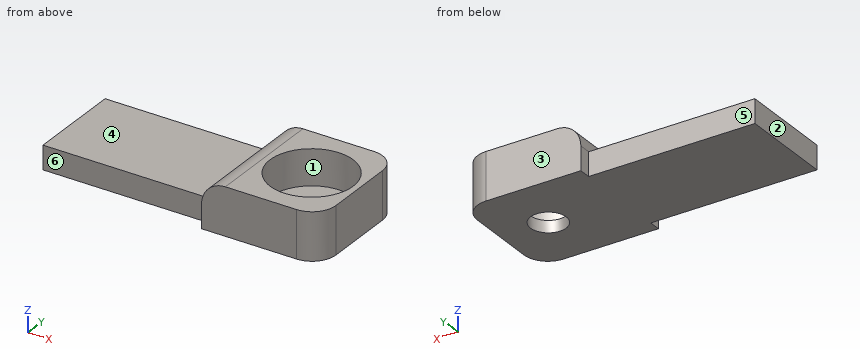
```python
from build123d import *

# Parameters (mm, degrees)
BOSS_EXTRUDE1_DEPTH = 20
CUT_EXTRUDE1_REACH  = 78.974
SKETCH2_R           = 7.5
SKETCH3_R           = 17.5
CUT_EXTRUDE2_DEPTH  = 15
SKETCH4_W           = 10
SKETCH4_H           = 40
CUT_EXTRUDE3_DEPTH  = 70
FILLET1_R           = 10
FILLET2_START       = -26
FILLET2_DEPTH       = 52


with BuildPart() as part:
    # Sketch1 → Boss-Extrude1 (new body)
    with BuildSketch(Plane.XY):
        Polygon((-70, 20), (0, 20), (0, 25), (50, 25), (50, -25), (0, -25), (0, -20), (-70, -20), align=None)
    extrude(amount=BOSS_EXTRUDE1_DEPTH)

    # Sketch2 → Cut-Extrude1 (cut, up to next)
    with BuildSketch(Plane.XY.offset(20), mode=Mode.PRIVATE) as cut_extrude1_sk1:
        with Locations((30, 0)):
            Circle(SKETCH2_R)
    cut_extrude1_tool1 = extrude(cut_extrude1_sk1.sketch, amount=-CUT_EXTRUDE1_REACH, mode=Mode.PRIVATE) & part.part
    add(cut_extrude1_tool1.solids().sort_by_distance((30, 0, 20))[0], mode=Mode.SUBTRACT)

    # Sketch3 → Cut-Extrude2 (cut)
    with BuildSketch(Plane.XY.offset(20)):
        with Locations((30, 0)):
            Circle(SKETCH3_R)
    extrude(amount=-CUT_EXTRUDE2_DEPTH, mode=Mode.SUBTRACT)

    # Sketch4 → Cut-Extrude3 (cut)
    with BuildSketch(Plane.ZY.offset(70)):
        with Locations((15, 0)):
            Rectangle(SKETCH4_W, SKETCH4_H)
    extrude(amount=-CUT_EXTRUDE3_DEPTH, mode=Mode.SUBTRACT)

    # Fillet1
    fillet1_edges = [part.edges().sort_by_distance(p)[0] for p in [
        (50, 25, 10),
        (50, -25, 10),
    ]]
    fillet(fillet1_edges, radius=FILLET1_R)

    # Fillet2: read off the stored shape, not the designer's step
    # Fillet2 outline → Fillet2 (cut)
    with BuildSketch(Plane(origin=(0, 0, 0), x_dir=(1, 0, 0), z_dir=(0, 1, 0)).offset(FILLET2_START)):
        with BuildLine():
            ThreePointArc((10, -20), (2.928932188, -17.071067812), (0, -10))
            Line((0, -10), (0, -20))
            Line((0, -20), (10, -20))
        make_face()
    extrude(amount=FILLET2_DEPTH, mode=Mode.SUBTRACT)


solid = part.part
```
Verification items for the finished model (mm, model axes). Face numbers are marked on the shaded views. A direction names the side the tool comes from. Give positions to 0.01 mm unless a question says otherwise; leave off trailing zeros. Order: outer loops, then holes, each group sorted by start corner. A loop starts at its lowest first (then second) coordinate and runs counter-clockwise, first axis right, second up. Notation, with made-up numbers: (21.25, 46.25) -> (58.25, 46.25) arc R23 ccw to (58.25, 67.25) -> close; hole circle Ø1 at (56, -16.75). An arc over 180 degrees is marked (long way). Use a Markdown table: item, result.
1) Tool access check on the marked faces 4, 5 and 6. Record the directions out of +Z, -Z, +X, -X, +Y, -Y that give a thin tool (end or side, any length) a straight path to the whole face; none if there is none.
Results:
| item | result |
|---|---|
| face 4 | +Z, -X, +Y, -Y |
| face 5 | +Z, -Z, -X, +Y |
| face 6 | +Z, -Z, -X, -Y |
2) Section check D-D, the plane x = 14.5. Record the boundary of the cut face in (y, z).
Results:
| item | result |
|---|---|
| outline | (-25, 0) -> (25, 0) -> (25, 20) -> (8.12, 20) -> (8.12, 5) -> (-8.12, 5) -> (-8.12, 20) -> (-25, 20) -> close |
3) Mould release check, pull along X, two halves, no side actions. Record for the marked faces 1, 2 and 3: pulls with the +X half, pulls with the -X half, needs draft (parallel to the pull), parting line crosses it, or undercut.
Results:
| item | result |
|---|---|
| face 1 | undercut |
| face 2 | pulls with the -X half |
| face 3 | needs draft |
4) Section check C-C, the plane x = 30. Record the boundary of the cut face in (y, z).
Results:
| item | result |
|---|---|
| outline | (-25, 0) -> (-7.5, 0) -> (-7.5, 5) -> (-17.5, 5) -> (-17.5, 20) -> (-25, 20) -> close; (7.5, 0) -> (25, 0) -> (25, 20) -> (17.5, 20) -> (17.5, 5) -> (7.5, 5) -> close |
5) Depth check by flat-ended pin: pin 1 Ø3 at (x, z) = (-46, 4) entering from +Y; pin 2 Ø1.5 at (y, z) = (-23, 4.5) entering from -X; pin 3 Ø19.5 at (x, y) = (30, 0) entering from +Z; pin 4 Ø8 at (x, z) = (-28, 16.5) entering from +Y. Enter the tip coordinate at first touch or a pass-through.
Results:
| item | result |
|---|---|
| pin 1 | y = 20 |
| pin 2 | x = 0 |
| pin 3 | z = 5 |
| pin 4 | through |
6) Section check B-B, the plane y = 0. Record the boundary of the cut face in (x, z).
Results:
| item | result |
|---|---|
| outline | (-70, 0) -> (22.5, 0) -> (22.5, 5) -> (12.5, 5) -> (12.5, 20) -> (10, 20) arc R10 ccw to (0, 10) -> (-70, 10) -> close; (37.5, 0) -> (50, 0) -> (50, 20) -> (47.5, 20) -> (47.5, 5) -> (37.5, 5) -> close |
7) Section check A-A, the plane z = 2.5. Record the boundary of the cut face in (x, y), then the cut area to 3 significant figures.
Results:
| item | result |
|---|---|
| outline | (-70, -20) -> (0, -20) -> (0, -25) -> (40, -25) arc R10 ccw to (50, -15) -> (50, 15) arc R10 ccw to (40, 25) -> (0, 25) -> (0, 20) -> (-70, 20) -> close; hole circle Ø15 at (30, 0) |
| area | 5,080 mm² |
8) Material ranges on probe 1 along Y at (x, z) = (30, 3.1); probe 2 along Y at (x, z) = (30, 14.25); probe 3 along Z at (x, y) = (-38, -0.5), recorded low to high.
Results:
| item | result |
|---|---|
| probe 1 | -25 to -7.5, 7.5 to 25 |
| probe 2 | -25 to -17.5, 17.5 to 25 |
| probe 3 | 0 to 10 |
